Could you check a few things on this model? Use its own coordinates, in mm. A direction names the side the tool comes from. Round coordinates to 2 decimals unless told otherwise and drop trailing zeros. Loops run counter-clockwise (first coordinate to the right, second up) from the corner with the lowest first, then second, coordinate; pieces in that order, holes last. Notation, with made-up numbers: (-35, 34.25) - (20, 34.25) arc R22 cw to (20, 66.25) - close; hole circle Ø2 at (6, 38.25). An arc over 180 degrees is marked (long way). Answer as CSV lines item,"result". Start each with the question number.
1) Which directions (+Z, -Z, +X, -X, +Y, -Y) give clear straight access to the entire face, cutting with the end or side of a thin tool? Please do faces 4 (the face through (7.6, 2.4, 6)), 5 (the face through (-0.33, 2.52, 16.1)).
2) Suppose I cut it at A-A, the plane x = 0. Write out the boundary of the cut face in (y, z), then the cut area to 3 significant figures.
3) Please list where these lines run through material, in increasing order: line 1 along Z through (x, y) = (4.5, 5.25); line 2 along Y through (x, z) = (0, 15); line 3 along Z through (x, y) = (-7.25, 7.5).
4) I'm going to push flat-ended pins straight in: pin 1 Ø3 at (y, z) = (8, 28) entering from -X; pin 2 Ø12 at (y, z) = (-2.5, 24) entering from -X; pin 3 Ø1.5 at (x, z) = (7.5, 26) entering from -Y. Where does each tip first touch, or does it pass through?
5) Suppose I cut it at D-D, the plane z = 19. Write out the boundary of the cut face in (x, y).
6) Suppose I cut it at C-C, the plane z = 30. Write out the boundary of the cut face in (x, y).
7) We'd pull the mould along Z, two halves only. Please class faces 1 (the face through (3, 0, 31.75)), 2 (the face through (-1.38, -6.2, 15.74)), 3 (the face through (3, 0, 0)): pulls with the +Z half, pulls with the -Z half, needs draft (parallel to the pull), parting line crosses it, or undercut.
```python
from build123d import *

# Parameters (mm, degrees)
F0_R     = 12.7
F1_DEPTH = 6.35
F2_R     = 6.35
F3_DEPTH = 25.4
F5_R     = 12.7
F6_DEPTH = 6.35
F7_R     = 2.54
F8_DEPTH = 31.75
F9_SIZE  = 5.08


# Not quite as in the source:
# - a pattern or mirror of a feature is missing from the dataset's text; its kind, count and spacing are read off the source's solid


with BuildPart() as f1:
    # F0 (on Top) → F1 (new body)
    with BuildSketch(Plane.XY):
        Circle(F0_R)
    extrude(amount=F1_DEPTH)


with BuildPart() as f1_copies_1:
    # F1_copies: instance of F1
    add(f1.part.mirror(Plane.XY.offset(15.875)))


with BuildPart() as f1_1:
    add(f1.part)

    add(f1_copies_1.part)  # F3 merges F1_copies_1
    # F2 (on Top) → F3 (join)
    with BuildSketch(Plane.XY):
        Circle(F2_R)
    extrude(amount=F3_DEPTH)

    # F5 (on face) → F6 (join)
    with BuildSketch(Plane.XY.offset(25.4)):
        Circle(F5_R)
    extrude(amount=F6_DEPTH)

    # F7 (on face) → F8 (cut)
    with BuildSketch(Plane.XY.offset(31.75)):
        Circle(F7_R)
    extrude(amount=-F8_DEPTH, mode=Mode.SUBTRACT)

    # F9
    f9_edges = [f1_1.edges().sort_by_distance(p)[0] for p in [
        (-12.7, 0, 25.4),
        (-12.7, 0, 6.35),
    ]]
    chamfer(f9_edges, length=F9_SIZE)


solid = f1_1.part
```
Filled sheet:
1,face 4,"none"
1,face 5,"+Z, -Z"
2,outline,"(-12.7, 0) - (-2.54, 0) - (-2.54, 31.75) - (-12.7, 31.75) - (-12.7, 30.48) - (-7.62, 25.4) - (-6.35, 25.4) - (-6.35, 6.35) - (-7.62, 6.35) - (-12.7, 1.27) - close; (2.54, 0) - (12.7, 0) - (12.7, 1.27) - (7.62, 6.35) - (6.35, 6.35) - (6.35, 25.4) - (7.62, 25.4) - (12.7, 30.48) - (12.7, 31.75) - (2.54, 31.75) - close"
2,area,"352 mm²"
3,line 1,"0 to 6.35, 25.4 to 31.75"
3,line 2,"-6.35 to -2.54, 2.54 to 6.35"
3,line 3,"0 to 3.54, 28.21 to 31.75"
4,pin 1,"x = -8.95"
4,pin 2,"x = -12.05"
4,pin 3,"y = -5.3"
5,outline,"circle Ø12.7 at (0, 0); hole circle Ø5.08 at (0, 0)"
6,outline,"circle Ø24.44 at (0, 0); hole circle Ø5.08 at (0, 0)"
7,face 1,"pulls with the +Z half"
7,face 2,"undercut"
7,face 3,"pulls with the -Z half"
